Check sheet for the modelled part. Datum: model origin and axes. Units: mm. A direction names the side the tool comes from. Give positions to 0.01 mm unless a question says otherwise; leave off trailing zeros. Loops run counter-clockwise (first coordinate to the right, second up) from the corner with the lowest first, then second, coordinate; pieces in that order, holes last. Notation, with made-up numbers: M 48,80 L 66,80 A37 ccw 66,119 Z; hole C 53,-2 d10. An arc over 180 degrees is marked long. Use one line per item in the form item = value.
from build123d import *

# Parameters (mm, degrees)
SKETCH008_W     = 149
SKETCH008_H     = 81.5
SKETCH008_R     = 4
SKETCH008_W_2   = 98.75
SKETCH008_H_2   = 57
PAD006_DEPTH    = 2
SKETCH009_W     = 15.9
SKETCH009_H     = 15.4
SKETCH009_W_2   = 13.5
SKETCH009_H_2   = 13
SKETCH009_W_3   = 110.15
SKETCH009_H_3   = 71.65
SKETCH009_W_4   = 107.75
SKETCH009_H_4   = 69.25
PAD007_DEPTH    = 5
SKETCH010_W     = 107.75
SKETCH010_H     = 69.25
SKETCH010_W_2   = 98.75
SKETCH010_H_2   = 57
PAD008_DEPTH    = 1
PAD009_DEPTH    = 6.55
SKETCH012_R     = 1.375
POCKET002_DEPTH = 4
SKETCH014_W     = 149
SKETCH014_H     = 81.5
SKETCH014_W_2   = 145
SKETCH014_H_2   = 77.5
PAD011_DEPTH    = 17
POCKET003_DEPTH = 98.75
POCKET004_DEPTH = 57


with BuildPart() as part:
    # Sketch008 (on Face27 of Binder) → Pad006 (new body)
    with BuildSketch(Plane.XY.offset(8.3)):
        with Locations((70.5, 36.75)):
            Rectangle(SKETCH008_W, SKETCH008_H)
        with Locations((131.5, 38.75)):
            Circle(SKETCH008_R, mode=Mode.SUBTRACT)
        with Locations((60.875, 39.25)):
            Rectangle(SKETCH008_W_2, SKETCH008_H_2, mode=Mode.SUBTRACT)
    extrude(amount=PAD006_DEPTH)

    # Sketch009 (on Face10 of Pad006) → Pad007 (join)
    with BuildSketch(Plane(origin=(0, 0, 8.3), x_dir=(1, 0, 0), z_dir=(0, 0, -1))):
        with Locations((131.5, -38.75)):
            Rectangle(SKETCH009_W, SKETCH009_H)
        with Locations((131.5, -38.75)):
            Rectangle(SKETCH009_W_2, SKETCH009_H_2, mode=Mode.SUBTRACT)
        with Locations((60.875, -36.875)):
            Rectangle(SKETCH009_W_3, SKETCH009_H_3)
        with Locations((60.875, -36.875)):
            Rectangle(SKETCH009_W_4, SKETCH009_H_4, mode=Mode.SUBTRACT)
    extrude(amount=PAD007_DEPTH)

    # Sketch010 (on Face4 of Pad007) → Pad008 (join)
    with BuildSketch(Plane(origin=(0, 0, 8.3), x_dir=(1, 0, 0), z_dir=(0, 0, -1))):
        with Locations((60.875, -36.875)):
            Rectangle(SKETCH010_W, SKETCH010_H)
        with Locations((60.875, -39.25)):
            Rectangle(SKETCH010_W_2, SKETCH010_H_2, mode=Mode.SUBTRACT)
    extrude(amount=PAD008_DEPTH)

    # Sketch011 (on Face4 of Pad008) → Pad009 (join)
    with BuildSketch(Plane(origin=(0, 0, 8.3), x_dir=(1, 0, 0), z_dir=(0, 0, -1))):
        with BuildLine():
            ThreePointArc((5.8, -0.996823), (-0.5835, -3.6665), (5.8, -6.336177))
            Line((5.8, -0.996823), (5.8, -6.336177))
        make_face()
        with BuildLine():
            ThreePointArc((5.8, -67.163823), (-0.5835, -69.8335), (5.8, -72.503177))
            Line((5.8, -67.163823), (5.8, -72.503177))
        make_face()
        with BuildLine():
            ThreePointArc((115.95, -72.76902), (122.0335, -69.8335), (115.95, -66.89798))
            Line((115.95, -72.76902), (115.95, -66.89798))
        make_face()
        with BuildLine():
            ThreePointArc((115.95, -6.60202), (122.0335, -3.6665), (115.95, -0.73098))
            Line((115.95, -0.73098), (115.95, -6.60202))
        make_face()
    extrude(amount=PAD009_DEPTH)

    # Sketch012 (on Face32 of Pad009) → Pocket002 (cut)
    with BuildSketch(Plane(origin=(0, 0, 1.75), x_dir=(1, 0, 0), z_dir=(0, 0, -1))):
        with Locations((118.2835, -3.6665)):
            Circle(SKETCH012_R)
        with Locations((118.2835, -69.8335)):
            Circle(SKETCH012_R)
        with Locations((3.1665, -69.8335)):
            Circle(SKETCH012_R)
        with Locations((3.1665, -3.6665)):
            Circle(SKETCH012_R)
    extrude(amount=-POCKET002_DEPTH, mode=Mode.SUBTRACT)

    # Sketch014 (on Face4 of Pocket002) → Pad011 (join)
    with BuildSketch(Plane(origin=(0, 0, 8.3), x_dir=(1, 0, 0), z_dir=(0, 0, -1))):
        with Locations((70.5, -36.75)):
            Rectangle(SKETCH014_W, SKETCH014_H)
        with Locations((70.5, -36.75)):
            Rectangle(SKETCH014_W_2, SKETCH014_H_2, mode=Mode.SUBTRACT)
    extrude(amount=PAD011_DEPTH)

    # Sketch015 (on Face10 of Pad011) → Pocket003 (cut)
    with BuildSketch(Plane.YZ.offset(11.5)):
        Polygon((67.75, 8.3), (67.75, 10.3), (69.150415, 10.3), align=None)
        Polygon((10.75, 8.3), (10.75, 10.3), (9.349585, 10.3), align=None)
    extrude(amount=POCKET003_DEPTH, mode=Mode.SUBTRACT)

    # Sketch016 (on Face28 of Pocket003) → Pocket004 (cut)
    with BuildSketch(Plane(origin=(0, 10.75, 0), x_dir=(-1, 0, 0), z_dir=(0, 1, 0))):
        Polygon((-110.25, 8.3), (-110.25, 10.3), (-111.650415, 10.3), align=None)
        Polygon((-11.5, 8.3), (-10.099585, 10.3), (-11.5, 10.3), align=None)
    extrude(amount=POCKET004_DEPTH, mode=Mode.SUBTRACT)

    # Sketch017 (on Face19 of Pocket004) → Groove (revolve, cut)
    with BuildSketch(Plane(origin=(0, 10.75, 0), x_dir=(-1, 0, 0), z_dir=(0, 1, 0))):
        Polygon((-110.25, 10.3), (-111.650415, 10.3), (-110.25, 8.3), align=None)
    revolve(axis=Axis((110.25, 10.75, 9.3), (0, 0, 1)), mode=Mode.SUBTRACT)

    # Sketch018 (on Face17 of Groove) → Groove001 (revolve, cut)
    with BuildSketch(Plane.XZ.offset(-67.75)):
        Polygon((111.650415, 10.3), (110.25, 10.3), (110.25, 8.3), align=None)
    revolve(axis=Axis((110.25, 67.75, 9.3), (0, 0, 1)), mode=Mode.SUBTRACT)

    # Sketch019 (on Face14 of Groove001) → Groove002 (revolve, cut)
    with BuildSketch(Plane.YZ.offset(11.5)):
        Polygon((67.75, 8.3), (69.150415, 10.3), (67.75, 10.3), align=None)
    revolve(axis=Axis((11.5, 67.75, 9.3), (0, 0, 1)), mode=Mode.SUBTRACT)

    # Sketch020 (on Face11 of Groove002) → Groove003 (revolve, cut)
    with BuildSketch(Plane(origin=(0, 10.75, 0), x_dir=(-1, 0, 0), z_dir=(0, 1, 0))):
        Polygon((-11.5, 8.3), (-10.099585, 10.3), (-11.5, 10.3), align=None)
    revolve(axis=Axis((11.5, 10.75, 9.3), (0, 0, -1)), mode=Mode.SUBTRACT)


solid = part.part
1) Depth check by flat-ended pin: pin 1 Ø2 at (x, y) = (3.17, 69.83) entering from -Z. Enter the tip coordinate at first touch or a pass-through.
Evaluation:
pin_1 = 5.75
2) Section check C-C (z = -6). Record the cut outline in (x, y), then the cut area to 3 significant figures.
Evaluation:
outline = M -4,-4 L 145,-4 L 145,77.5 L -4,77.5 Z; hole M -2,-2 L 143,-2 L 143,75.5 L -2,75.5 Z
area = 906 mm^2
3) Section check D-D (y = 29). Record the cut outline in (x, z).
Evaluation:
outline = M -4,-8.7 L -2,-8.7 L -2,8.3 L 5.8,8.3 L 5.8,3.3 L 7,3.3 L 7,7.3 L 11.5,7.3 L 11.5,8.3 L 10.1,10.3 L -4,10.3 Z; M 110.25,7.3 L 114.75,7.3 L 114.75,3.3 L 115.95,3.3 L 115.95,8.3 L 143,8.3 L 143,-8.7 L 145,-8.7 L 145,10.3 L 111.65,10.3 L 110.25,8.3 Z
4) Section check A-A (x = 65). Record the cut outline in (y, z), then the cut area to 3 significant figures.
Evaluation:
outline = M -4,-8.7 L -2,-8.7 L -2,8.3 L 1.05,8.3 L 1.05,3.3 L 2.25,3.3 L 2.25,7.3 L 10.75,7.3 L 10.75,8.3 L 9.35,10.3 L -4,10.3 Z; M 67.75,7.3 L 71.5,7.3 L 71.5,3.3 L 72.7,3.3 L 72.7,8.3 L 75.5,8.3 L 75.5,-8.7 L 77.5,-8.7 L 77.5,10.3 L 69.15,10.3 L 67.75,8.3 Z
area = 138 mm^2
5) Release check for a two-part mould opening along X. For faces 3 (the face through (143, 37, 0)), 4 (the face through (-4, 37, 1)), 5 (the face through (70, 76, -8.7)) record: pulls with the +X half, pulls with the -X half, needs draft (parallel to the pull), parting line crosses it, or undercut.
Evaluation:
face_3 = undercut
face_4 = pulls with the -X half
face_5 = needs draft
6) Set-up check for faces 1 (the face through (60, 2.25, 5)), 2 (the face through (145, 37, 1)): record each of +Z, -Z, +X, -X, +Y, -Y from which the full face is reachable in a straight line by a thin tool's end or side.
Evaluation:
face_1 = -Z
face_2 = +Z, -Z, +X, +Y, -Y
7) Scan lines: line 1 (X direction, y = 63.5, z = 7.5); line 2 (X direction, y = 59.5, z = 5.75); line 3 (X direction, y = 5.5, z = -5). Record each from-to range of solid material in increasing order.
Evaluation:
line_1 = -4 to -2, 5.8 to 11.5, 110.25 to 115.95, 143 to 145
line_2 = -4 to -2, 5.8 to 7, 114.75 to 115.95, 143 to 145
line_3 = -4 to -2, 143 to 145
8) Section check B-B (y = 38.75). State how many separate pieces and enclosed holes the cut face has, then the cut area to 3 significant figures.
Evaluation:
separate_pieces = 3
enclosed_holes = 0
area = 183 mm^2
